from build123d import *

# Parameters (mm, degrees)
SKETCH1_W                 = 190.5
SKETCH1_H                 = 139.7
BOSS_EXTRUDE1_DEPTH       = 6.35
SKETCH13_W                = 25.4
SKETCH13_H                = 6.35
CUT_EXTRUDE6_DEPTH        = 6.35
LPATTERN7_COUNT           = 2
LPATTERN7_PITCH           = 120.65
SKETCH14_W                = 6.35
SKETCH14_H                = 25.4
CUT_EXTRUDE7_DEPTH        = 6.35
F_8_CLEARANCE_HOLE1_D     = 4.4958
F_8_CLEARANCE_HOLE1_DEPTH = 10.16
F_8_CLEARANCE_HOLE1_TIP   = 1.350674586
SKETCH18_R                = 14.2875
CUT_EXTRUDE9_DEPTH        = 7.62
CUT_EXTRUDE16_DEPTH       = 6.35
FILLET2_R                 = 0.508
CUT_EXTRUDE17_DEPTH       = 6.35
FILLET5_R                 = 0.508
FILLET6_R                 = 12.7


with BuildPart() as part:
    # Sketch1 → Boss-Extrude1 (new body)
    with BuildSketch(Plane(origin=(0, 0, 0), x_dir=(1, 0, 0), z_dir=(0, 1, 0))):
        with Locations((95.25, 69.85)):
            Rectangle(SKETCH1_W, SKETCH1_H)
    extrude(amount=BOSS_EXTRUDE1_DEPTH)

    # Sketch13 → Cut-Extrude6 (cut)
    with BuildSketch(Plane(origin=(0, 6.35, 0), x_dir=(1, 0, 0), z_dir=(0, 1, 0))):
        with Locations((44.45, 9.525)):
            Rectangle(SKETCH13_W, SKETCH13_H)
        with Locations((95.25, 9.525)):
            Rectangle(SKETCH13_W, SKETCH13_H)
        with Locations((146.05, 9.525)):
            Rectangle(SKETCH13_W, SKETCH13_H)
    cut_extrude6 = extrude(amount=-CUT_EXTRUDE6_DEPTH, mode=Mode.SUBTRACT)

    # LPattern7: Cut-Extrude6 ×2
    with Locations(*[(0, 0, -i * LPATTERN7_PITCH) for i in range(1, LPATTERN7_COUNT)]):
        add(cut_extrude6, mode=Mode.SUBTRACT)

    # Sketch14 → Cut-Extrude7 (cut)
    with BuildSketch(Plane(origin=(0, 6.35, 0), x_dir=(1, 0, 0), z_dir=(0, 1, 0))):
        with Locations((9.525, 44.45)):
            Rectangle(SKETCH14_W, SKETCH14_H)
        with Locations((180.975, 44.45)):
            Rectangle(SKETCH14_W, SKETCH14_H)
        with Locations((180.975, 95.25)):
            Rectangle(SKETCH14_W, SKETCH14_H)
        with Locations((9.525, 95.25)):
            Rectangle(SKETCH14_W, SKETCH14_H)
    extrude(amount=-CUT_EXTRUDE7_DEPTH, mode=Mode.SUBTRACT)

    # #8 Clearance Hole1
    with Locations(Plane(origin=(0, 6.35, 0), x_dir=(1, 0, 0), z_dir=(0, 1, 0))):
        with Locations((9.525, 69.85), (180.975, 69.85)):
            Hole(F_8_CLEARANCE_HOLE1_D / 2, depth=F_8_CLEARANCE_HOLE1_DEPTH)
            with Locations((0, 0, -(F_8_CLEARANCE_HOLE1_DEPTH + F_8_CLEARANCE_HOLE1_TIP / 2))):  # 118° drill point
                Cone(0, F_8_CLEARANCE_HOLE1_D / 2, F_8_CLEARANCE_HOLE1_TIP, mode=Mode.SUBTRACT)

    # Sketch18 → Cut-Extrude9 (cut)
    with BuildSketch(Plane(origin=(0, 6.35, 0), x_dir=(1, 0, 0), z_dir=(0, 1, 0))):
        with Locations(Location((95.25, 69.85, 0), (0, 0, 270))):
            Circle(SKETCH18_R)
    extrude(amount=-CUT_EXTRUDE9_DEPTH, mode=Mode.SUBTRACT)

    # Sketch24 → Cut-Extrude16 (cut)
    with BuildSketch(Plane(origin=(0, 6.35, 0), x_dir=(1, 0, 0), z_dir=(0, 1, 0))):
        with BuildLine():
            Line((34.925, 87.63), (34.925, 69.85))
            ThreePointArc((34.925, 69.85), (47.625, 57.15), (60.325, 69.85))
            Line((60.325, 69.85), (60.325, 87.63))
            Line((60.325, 87.63), (52.902309744, 81.401623344))
            ThreePointArc((52.902309744, 81.401623344), (47.625, 82.55), (42.347690256, 81.401623344))
            Line((42.347690256, 81.401623344), (34.925, 87.63))
        make_face()
    extrude(amount=-CUT_EXTRUDE16_DEPTH, mode=Mode.SUBTRACT)

    # Fillet2
    fillet2_edges = [part.edges().sort_by_distance(p)[0] for p in [
        (34.925, 3.175, -87.63),
        (42.347690256, 3.175, -81.401623344),
        (52.902309744, 3.175, -81.401623344),
        (60.325, 3.175, -87.63),
    ]]
    fillet(fillet2_edges, radius=FILLET2_R)

    # Sketch25 → Cut-Extrude17 (cut)
    with BuildSketch(Plane(origin=(0, 6.35, 0), x_dir=(1, 0, 0), z_dir=(0, 1, 0))):
        with BuildLine():
            ThreePointArc((135.255, 80.01), (131.515774674, 75.529612663), (130.175, 69.85))
            ThreePointArc((130.175, 69.85), (130.178809834, 69.538944895), (130.190237052, 69.228076416))
            ThreePointArc((130.190237052, 69.228076416), (142.875, 57.15), (155.559762948, 69.228076416))
            ThreePointArc((155.559762948, 69.228076416), (155.571190166, 69.538944895), (155.575, 69.85))
            ThreePointArc((155.575, 69.85), (154.234225326, 75.529612663), (150.495, 80.01))
            ThreePointArc((150.495, 80.01), (149.361085379, 80.768823035), (148.152309744, 81.401623344))
            ThreePointArc((148.152309744, 81.401623344), (142.875, 82.55), (137.597690256, 81.401623344))
            ThreePointArc((137.597690256, 81.401623344), (136.388914621, 80.768823035), (135.255, 80.01))
        make_face()
        with BuildLine():
            Line((137.597690256, 81.401623344), (130.175, 87.63))
            Line((130.175, 87.63), (130.175, 69.85))
            ThreePointArc((130.175, 69.85), (131.515774674, 75.529612663), (135.255, 80.01))
            ThreePointArc((135.255, 80.01), (136.388914621, 80.768823035), (137.597690256, 81.401623344))
        make_face()
        with BuildLine():
            Line((155.575, 87.63), (148.152309744, 81.401623344))
            ThreePointArc((148.152309744, 81.401623344), (149.361085379, 80.768823035), (150.495, 80.01))
            ThreePointArc((150.495, 80.01), (154.234225326, 75.529612663), (155.575, 69.85))
            Line((155.575, 69.85), (155.575, 87.63))
        make_face()
    extrude(amount=-CUT_EXTRUDE17_DEPTH, mode=Mode.SUBTRACT)

    # Fillet5
    fillet5_edges = [part.edges().sort_by_distance(p)[0] for p in [
        (130.175, 3.175, -87.63),
        (137.597690256, 3.175, -81.401623344),
        (148.152309744, 3.175, -81.401623344),
        (155.575, 3.175, -87.63),
    ]]
    fillet(fillet5_edges, radius=FILLET5_R)

    # Fillet6
    fillet6_edges = [part.edges().sort_by_distance(p)[0] for p in [
        (0, 3.175, -139.7),
        (190.5, 3.175, -139.7),
        (190.5, 3.175, 0),
        (0, 3.175, 0),
    ]]
    fillet(fillet6_edges, radius=FILLET6_R)


solid = part.part
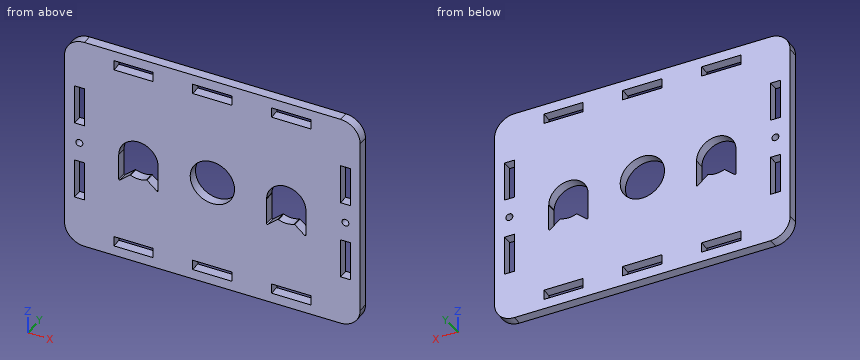
Geometry: final body of the model. Coordinates: model frame, mm. Round coordinates to 2 decimals unless told otherwise and drop trailing zeros. Order: outer loops, then holes, each group sorted by start corner. A loop starts at its lowest first (then second) coordinate and runs counter-clockwise, first axis right, second up. Notation, with made-up numbers: (0, 38) -> (53, 38) arc R14 ccw to (53, 44) -> close; hole circle Ø3 at (62, -29). An arc over 180 degrees is marked (long way). Put each result on its own line as item: value. Start each with the question number.
Q1. Line query: probe 1 along X at (y, z) = (5.75, -37); probe 2 along X at (y, z) = (3, -69.85) (1 decimal); probe 3 along Z at (x, y) = (135.5, 0.5). Output: solid intervals per line, ascending.
Q2. Section D-D on y = 3. Give the number of separate pieces and of enclosed holes in the cut face, and give its area (3 significant figures).
Q3. Section B-B on x = 95.25. Return the cut outline in (y, z).
Q4. Section C-C on z = -61.5. Return the cut outline in (x, y), and give its area (3 significant figures).
Q5. First-contact query: pin 1 (3 mm diameter, centred on y = 3.5, z = -10, fed in from +X); pin 2 (1.9 mm diameter, centred on y = 3.5, z = -8, fed in from -X); pin 3 (10 mm diameter, centred on x = 117.5, z = -38.5, fed in from -Y); pin 4 (3 mm diameter, centred on y = 2.5, z = -131.5, fed in from +X). Flat tips, straight axial feed; report the tip coordinate or a pass-through.
Q6. Section A-A on z = -101.5. Return the cut outline in (x, y), and give its area (3 significant figures).
Ans:
1. probe 1: x = 0 to 6.35, 12.7 to 177.8, 184.15 to 190.5
1. probe 2: x = 0 to 7.3, 11.8 to 34.9, 60.3 to 81, 109.5 to 130.2, 155.6 to 178.7, 183.2 to 190.5
1. probe 3: z = -139.7 to -133.35, -127 to -83.16, -59.51 to -12.7, -6.35 to 0
2. separate pieces: 1
2. enclosed holes: 15
2. area: 23,000 mm2
3. outline: (0, -139.7) -> (6.35, -139.7) -> (6.35, -133.35) -> (0, -133.35) -> close; (0, -127) -> (6.35, -127) -> (6.35, -84.14) -> (0, -84.14) -> close; (0, -55.56) -> (6.35, -55.56) -> (6.35, -12.7) -> (0, -12.7) -> close; (0, -6.35) -> (6.35, -6.35) -> (6.35, 0) -> (0, 0) -> close
4. outline: (0, 0) -> (38.06, 0) -> (38.06, 6.35) -> (0, 6.35) -> close; (57.19, 0) -> (83.66, 0) -> (83.66, 6.35) -> (57.19, 6.35) -> close; (106.84, 0) -> (133.31, 0) -> (133.31, 6.35) -> (106.84, 6.35) -> close; (152.44, 0) -> (190.5, 0) -> (190.5, 6.35) -> (152.44, 6.35) -> close
4. area: 819 mm2
5. pin 1: stops at x = 190.44
5. pin 2: stops at x = 0.57
5. pin 3: stops at y = 0
5. pin 4: stops at x = 190.14
6. outline: (0, 0) -> (6.35, 0) -> (6.35, 6.35) -> (0, 6.35) -> close; (12.7, 0) -> (177.8, 0) -> (177.8, 6.35) -> (12.7, 6.35) -> close; (184.15, 0) -> (190.5, 0) -> (190.5, 6.35) -> (184.15, 6.35) -> close
6. area: 1,130 mm2
